The figure shows three views and two pictorial views of one solid part (mm, origin at its lowest corner). Answer the questions. A direction names the side the tool comes from. Round coordinates to 2 decimals unless told otherwise and drop trailing zeros. Write each loop counter-clockwise with the first axis right and the second up, starting at its lowest first coordinate (ties: lowest second). Pieces come first, ordered by that corner, then holes. Notation, with made-up numbers: (-31.5, 25.5) - (-0.5, 25.5) arc R24 cw to (-0.5, 57.5) - close; hole circle Ø8 at (-35.75, 52). An arc over 180 degrees is marked (long way). Answer as CSV lines item,"result". Start each with the question number.
Item 1: A cutting plane is placed at A-A on y = 73. State how many separate pieces and enclosed holes the cut face has, and give its area (4 significant figures).
Item 2: A cutting plane is placed at C-C on x = 136. Determine the outline of the cut face in (y, z) (1 decimal).
Item 3: Straight lines are drawn through the part: line 1 along X through (y, z) = (56, 10.25) (1 decimal); line 2 along X through (y, z) = (105, 18) (1 decimal); line 3 along X through (y, z) = (39, 27.25). For each, find the intervals that lie inside material, in ascending order. Write a range as [from, to].
Item 4: Which of the six approach directions +Z, -Z, +X, -X, +Y, -Y give full straight-line access (tool end or side, diameter ignored) to the marked faces 1, 2 and 3?
Item 5: Flat-ended cylindrical pins translate along their axes: pin 1 (5.5 mm diameter, centred on x = 215.9, z = 14.29, fed in from -Y); pin 2 (8.5 mm diameter, centred on x = 96, z = 13, fed in from -Y); pin 3 (14.5 mm diameter, centred on y = 31.5, z = 13.5, fed in from -X); pin 4 (12 mm diameter, centred on y = 77.5, z = 13.5, fed in from +X). Find the tip coordinate at first contact, or state that the pin passes through.
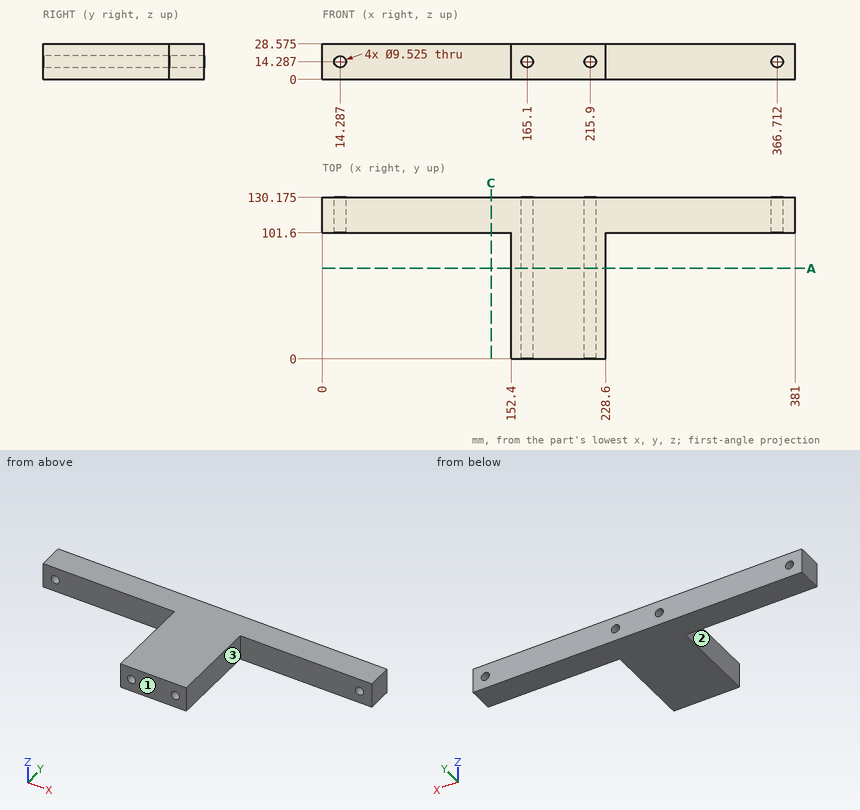
Geometry says:
1,separate pieces,"1"
1,enclosed holes,"2"
1,area,"2,035 mm^2"
2,outline,"(101.6, 0) - (130.2, 0) - (130.2, 28.6) - (101.6, 28.6) - close"
3,line 1,"x = [152.4, 162.6], [167.6, 213.4], [218.4, 228.6]"
3,line 2,"x = [0, 11.3], [17.3, 162.1], [168.1, 212.9], [218.9, 363.7], [369.7, 381]"
3,line 3,"x = [152.4, 228.6]"
4,face 1,"+Z, -Z, +X, -X, -Y"
4,face 2,"+Z, -Z, -X, -Y"
4,face 3,"+Z, -Z, +X, -Y"
5,pin 1,"passes through"
5,pin 2,"stops at y = 101.6"
5,pin 3,"stops at x = 152.4"
5,pin 4,"stops at x = 228.6"
